```python
from build123d import *

# Parameters (mm, degrees)
F1_DEPTH = 147.6375
F0_W     = 588.575
F0_H     = 11.9
F2_DEPTH = 146.84375


with BuildPart() as f1:
    # F0 (on Front) → F1 (new body, symmetric)
    with BuildSketch(Plane.XZ):
        Polygon((-306.3875, 295.275), (-306.3875, 0), (-294.2875, 0), (-294.2875, 136.425), (-294.2875, 148.325), (-294.2875, 281.075), (-294.2875, 292.975), (-294.2875, 295.275), align=None)
        Polygon((294.2875, 148.325), (294.2875, 136.425), (294.2875, 0), (306.3875, 0), (306.3875, 295.275), (294.2875, 295.275), (294.2875, 292.975), (294.2875, 281.075), align=None)
    extrude(amount=F1_DEPTH, both=True)

    # F0 (on Front) → F2 (join, symmetric)
    with BuildSketch(Plane.XZ):
        with Locations((0, 287.025)):
            Rectangle(F0_W, F0_H)
        with Locations((0, 142.375)):
            Rectangle(F0_W, F0_H)
    extrude(amount=F2_DEPTH, both=True)


solid = f1.part
```
Input: part model. Units: mm. Frame: model coordinates. A direction names the side the tool comes from. Give positions to 0.01 mm unless a question says otherwise; leave off trailing zeros. Write each loop counter-clockwise with the first axis right and the second up, starting at its lowest first coordinate (ties: lowest second). Pieces come first, ordered by that corner, then holes. Notation, with made-up numbers: (1, 83.5) - (29, 83.5) arc R12 cw to (29, 99.5) - close; hole circle Ø11 at (22, 29.25). An arc over 180 degrees is marked (long way). Write item = value, one per line. Start each with the question number.
1) Cut plane B-B (y = 100). Return loops of the section in (x, z) (1 decimal).
2) Reachability of faces 4 (the face through (-4, -146.844, 287)), 5 (the face through (-4, -2, 148.325)), 6 (the face through (-4, 2, 292.975)), 7 (the face through (-4, -2, 136.425)) from +Z, -Z, +X, -X, +Y, -Y: full face, straight path, thin tool, end or side. Return the list, or none.
3) Cut plane A-A (x = 104). Return loops of the section in (y, z) (3 decimals).
4) Draft query along Z for faces 1 (the face through (-4, 146.844, 287)), 2 (the face through (-4, 2, 281.075)), 3 (the face through (300, -2, 0)). Return one class per face: pulls with the +Z half, pulls with the -Z half, needs draft (parallel to the pull), parting line crosses it, or undercut.
5) Pin query (flat end, axial travel): pin 1 (5 mm diameter, centred on x = 34.5, y = -72.5, fed in from -Z) (3 decimals); pin 2 (6 mm diameter, centred on x = 62, z = 143, fed in from +Y); pin 3 (3 mm diameter, centred on x = 132.5, y = 39, fed in from +Z) (3 decimals). Return the tip coordinate at first contact, or that it passes through.
6) Cut plane C-C (z = 214). Return loops of the section in (x, y), and give its area (3 significant figures).
7) Material intervals for L1, parallel to X at y = 128, z = 213.5; L2, parallel to Z at x = 108, y = 92 (3 decimals); L3, parallel to Y at x = -133.5, z = 145, sorted ascending. Write a range as [from, to].
Answers follow:
q1.outline = (-306.4, 0) - (-294.3, 0) - (-294.3, 136.4) - (294.3, 136.4) - (294.3, 0) - (306.4, 0) - (306.4, 295.3) - (294.3, 295.3) - (294.3, 293) - (-294.3, 293) - (-294.3, 295.3) - (-306.4, 295.3) - close; hole (-294.3, 148.3) - (294.3, 148.3) - (294.3, 281.1) - (-294.3, 281.1) - close
q2.face_4 = +Z, -Z, -Y
q2.face_5 = +Y, -Y
q2.face_6 = +Z, +Y, -Y
q2.face_7 = -Z, +Y, -Y
q3.outline = (-146.844, 136.425) - (146.844, 136.425) - (146.844, 148.325) - (-146.844, 148.325) - close; (-146.844, 281.075) - (146.844, 281.075) - (146.844, 292.975) - (-146.844, 292.975) - close
q4.face_1 = needs draft
q4.face_2 = undercut
q4.face_3 = pulls with the -Z half
q5.pin_1 = 136.425
q5.pin_2 = 146.84
q5.pin_3 = 292.975
q6.outline = (-306.39, -147.64) - (-294.29, -147.64) - (-294.29, 147.64) - (-306.39, 147.64) - close; (294.29, -147.64) - (306.39, -147.64) - (306.39, 147.64) - (294.29, 147.64) - close
q6.area = 7,150 mm^2
q7.L1 = [-306.39, -294.29], [294.29, 306.39]
q7.L2 = [136.425, 148.325], [281.075, 292.975]
q7.L3 = [-146.84, 146.84]
